from build123d import *

# Parameters (mm, degrees)
ESQUISSE1_R          = 30
ESQUISSE1_R_2        = 19
BOSS_EXTRU_1_DEPTH   = 20
EMPREINTE1_OUTLINE_R = 19
EMPREINTE1_DEPTH     = 20


# Read off the part's stored shape, not the designer's step: Empreinte1
with BuildPart() as part:
    # Esquisse1 → Boss.-Extru.1 (new body)
    with BuildSketch(Plane(origin=(0, 0, 0), x_dir=(1, 0, 0), z_dir=(0, 1, 0))):
        with Locations(Location((0, 0, 0), (0, 0, 270))):
            Circle(ESQUISSE1_R)
        with Locations(Location((0, 0, 0), (0, 0, 270))):
            Circle(ESQUISSE1_R_2, mode=Mode.SUBTRACT)
    extrude(amount=BOSS_EXTRU_1_DEPTH)

    # Empreinte1 outline → Empreinte1 (cut)
    with BuildSketch(Plane(origin=(0, 0, 0), x_dir=(1, 0, 0), z_dir=(0, 1, 0))):
        with BuildLine():
            ThreePointArc((-12.25, 21.217622393), (-10.200961894, 20.668584287), (-10.75, 18.619546181))
            ThreePointArc((-10.75, 18.619546181), (-18.619546181, 10.75), (-21.5, 0))
            ThreePointArc((-21.5, 0), (-23, -1.5), (-24.5, 0))
            ThreePointArc((-24.5, 0), (-24.290399104, 3.197891709), (-23.665182744, 6.341066605))
            ThreePointArc((-23.665182744, 6.341066605), (-24.725842916, 8.178183912), (-26.562960223, 7.11752374))
            ThreePointArc((-26.562960223, 7.11752374), (-23.815698604, -13.75), (-7.11752374, -26.562960223))
            ThreePointArc((-7.11752374, -26.562960223), (-5.280406433, -25.502300051), (-6.341066605, -23.665182744))
            ThreePointArc((-6.341066605, -23.665182744), (-9.375744093, -22.635048547), (-12.25, -21.217622393))
            ThreePointArc((-12.25, -21.217622393), (-12.799038106, -19.168584287), (-10.75, -18.619546181))
            ThreePointArc((-10.75, -18.619546181), (0, -21.5), (10.75, -18.619546181))
            ThreePointArc((10.75, -18.619546181), (12.799038106, -19.168584287), (12.25, -21.217622393))
            ThreePointArc((12.25, -21.217622393), (9.375744093, -22.635048547), (6.341066605, -23.665182744))
            ThreePointArc((6.341066605, -23.665182744), (5.280406433, -25.502300051), (7.11752374, -26.562960223))
            ThreePointArc((7.11752374, -26.562960223), (23.815698604, -13.75), (26.562960223, 7.11752374))
            ThreePointArc((26.562960223, 7.11752374), (24.725842916, 8.178183912), (23.665182744, 6.341066605))
            ThreePointArc((23.665182744, 6.341066605), (24.290399104, 3.197891709), (24.5, 0))
            ThreePointArc((24.5, 0), (23, -1.5), (21.5, 0))
            ThreePointArc((21.5, 0), (18.619546181, 10.75), (10.75, 18.619546181))
            ThreePointArc((10.75, 18.619546181), (10.200961894, 20.668584287), (12.25, 21.217622393))
            ThreePointArc((12.25, 21.217622393), (14.914655011, 19.437156837), (17.324116139, 17.324116139))
            ThreePointArc((17.324116139, 17.324116139), (19.445436483, 17.324116139), (19.445436483, 19.445436483))
            ThreePointArc((19.445436483, 19.445436483), (0, 27.5), (-19.445436483, 19.445436483))
            ThreePointArc((-19.445436483, 19.445436483), (-19.445436483, 17.324116139), (-17.324116139, 17.324116139))
            ThreePointArc((-17.324116139, 17.324116139), (-14.914655011, 19.437156837), (-12.25, 21.217622393))
        make_face()
        Circle(EMPREINTE1_OUTLINE_R, mode=Mode.SUBTRACT)
    extrude(amount=EMPREINTE1_DEPTH, mode=Mode.SUBTRACT)


solid = part.part
Input: part model. Units: mm. Frame: model coordinates. A direction names the side the tool comes from. Give positions to 0.01 mm unless a question says otherwise; leave off trailing zeros. Loops run counter-clockwise (first coordinate to the right, second up) from the corner with the lowest first, then second, coordinate; pieces in that order, holes last. Notation, with made-up numbers: (65, 88) - (123, 88) arc R19 ccw to (123, 117) - close; hole circle Ø9 at (54, -26). An arc over 180 degrees is marked (long way). Use CSV: the item, a comma, the result in double quotes. Start each with the question number.
Item 1: Section D-D on x = -15.5. Return loops of the section in (y, z), then the cut area to 3 significant figures.
Item 2: Reachability of faces 1 (the cylindrical face through (-14.95, 9.86, -19.41)), 2 (the flat face through (-20, 20, -9)) from +Z, -Z, +X, -X, +Y, -Y: full face, straight path, thin tool, end or side. Return the list, or none.
Item 3: Mould query, pull axis Z, two halves, no side actions, for faces 3 (the flat face through (-20, 0, -9)), 4 (the cylindrical face through (-18.54, 9.86, -10.89)), 5 (the cylindrical face through (1.32, 9.86, -29.97)). Classes: pulls with the +Z half, pulls with the -Z half, needs draft (parallel to the pull), parting line crosses it, or undercut.
Item 4: Section B-B on y = 8. Return loops of the section in (x, z).
Item 5: Section A-A on x = 0. Return loops of the section in (y, z).
Item 6: Contact query for flat-ended pins moving along their axis: P1, Ø12, axis at y = 15.5, z = -12.5, coming from the +X side; P2, Ø10, axis at x = 20.5, y = 17.5, coming from the +Z side; P3, Ø3, axis at x = 10, y = 12, coming from the -Z side. Output: stop coordinate, or through.
Item 7: Line query: line 1 (Z direction, x = 5.5, y = 5.25); line 2 (X direction, y = 8.5, z = -20); line 3 (Z direction, x = -16, y = 11.75). Output: solid intervals per line, ascending.
Item 8: Section C-C on z = -5. Return loops of the section in (x, y), then the cut area to 3 significant figures.
Ans:
1,outline,"(0, -25.69) - (20, -25.69) - (20, -22.72) - (0, -22.72) - close; (0, -18.97) - (20, -18.97) - (20, -14.9) - (0, -14.9) - close; (0, 22.72) - (20, 22.72) - (20, 25.69) - (0, 25.69) - close"
1,area,"200 mm2"
2,face 1,"+Y, -Y"
2,face 2,"+Z, -Z, +X, -X, +Y"
3,face 3,"needs draft"
3,face 4,"undercut"
3,face 5,"parting line crosses it"
4,outline,"circle Ø60 at (0, 0); hole (-26.56, -7.12) arc R1.5 ccw to (-23.67, -6.34) arc R24.5 cw to (-24.5, 0) arc R1.5 cw to (-21.5, 0) arc R21.5 ccw to (-10.75, -18.62) arc R1.5 cw to (-12.25, -21.22) arc R24.5 cw to (-17.32, -17.32) arc R1.5 ccw to (-19.45, -19.45) arc R27.5 ccw to (19.45, -19.45) arc R1.5 ccw to (17.32, -17.32) arc R24.5 cw to (12.25, -21.22) arc R1.5 cw to (10.75, -18.62) arc R21.5 ccw to (21.5, 0) arc R1.5 cw to (24.5, 0) arc R24.5 cw to (23.67, -6.34) arc R1.5 ccw to (26.56, -7.12) arc R27.5 ccw to (7.12, 26.56) arc R1.5 ccw to (6.34, 23.67) arc R24.5 cw to (12.25, 21.22) arc R1.5 cw to (10.75, 18.62) arc R21.5 ccw to (-10.75, 18.62) arc R1.5 cw to (-12.25, 21.22) arc R24.5 cw to (-6.34, 23.67) arc R1.5 ccw to (-7.12, 26.56) arc R27.5 ccw to start"
5,outline,"(0, -30) - (20, -30) - (20, -27.5) - (0, -27.5) - close; (0, 21.5) - (20, 21.5) - (20, 30) - (0, 30) - close"
6,P1,"stops at x = 29.29"
6,P2,"stops at z = 25.69"
6,P3,"stops at z = -28.77"
7,line 1,"z = -29.49 to -26.94, 20.78 to 24.25, 25.97 to 29.49"
7,line 2,"x = -22.36 to -18.87, -14.15 to -10, 10 to 14.15, 18.87 to 22.36"
7,line 3,"z = -25.38 to -22.37, -18.55 to -14.36, 22.37 to 25.38"
8,outline,"(-29.58, 0) - (-27.04, 0) - (-27.04, 20) - (-29.58, 20) - close; (-23.98, 0) - (-20.91, 0) - (-20.91, 20) - (-23.98, 20) - close; (20.91, 0) - (23.98, 0) - (23.98, 20) - (20.91, 20) - close; (27.04, 0) - (29.58, 0) - (29.58, 20) - (27.04, 20) - close"
8,area,"225 mm2"
